```python
from build123d import *

# Parameters (mm, degrees)
BOSS_EXTRUDE1_DEPTH                    = 44
CBORE_FOR_M8_HEX_HEAD_BOLT1_AT_2_COUNT = 2
CBORE_FOR_M8_HEX_HEAD_BOLT1_AT_2_PITCH = 52
CBORE_FOR_M8_HEX_HEAD_BOLT1_AT_3_COUNT = 2
CBORE_FOR_M8_HEX_HEAD_BOLT1_AT_3_PITCH = 71.4177849
CBORE_FOR_M8_HEX_HEAD_BOLT1_AT_4_COUNT = 2
CBORE_FOR_M8_HEX_HEAD_BOLT1_AT_4_PITCH = 101
CBORE_FOR_M8_HEX_HEAD_BOLT1_AT_5_COUNT = 2
CBORE_FOR_M8_HEX_HEAD_BOLT1_AT_5_PITCH = 86.585218138
CBORE_FOR_M8_HEX_HEAD_BOLT1_AT_6_COUNT = 2
CBORE_FOR_M8_HEX_HEAD_BOLT1_AT_6_PITCH = 71.4177849
SKETCH9_W                              = 236.92276851
SKETCH9_H                              = 228.212372608
CUT_EXTRUDE1_DEPTH                     = 10
SKETCH8_R                              = 6
CUT_EXTRUDE2_DEPTH                     = 139.585713549


with BuildPart() as part:
    # Sketch1 → Boss-Extrude1 (new body)
    with BuildSketch(Plane(origin=(0, 0, 0), x_dir=(1, 0, 0), z_dir=(0, 1, 0))):
        with BuildLine():
            Line((77.338541491, -95), (-77.338541491, -95))
            ThreePointArc((-77.338541491, -95), (-86.620580695, -86.620580695), (-95, -77.338541491))
            Line((-95, -77.338541491), (-95, 77.338541491))
            ThreePointArc((-95, 77.338541491), (-86.620580695, 86.620580695), (-77.338541491, 95))
            Line((-77.338541491, 95), (77.338541491, 95))
            ThreePointArc((77.338541491, 95), (86.620580695, 86.620580695), (95, 77.338541491))
            Line((95, 77.338541491), (95, -77.338541491))
            ThreePointArc((95, -77.338541491), (86.620580695, -86.620580695), (77.338541491, -95))
        make_face()
    extrude(amount=BOSS_EXTRUDE1_DEPTH)

    # Sketch2 → Cut-Revolve3 (revolve, cut)
    with BuildSketch(Plane(origin=(0, 0, 0), x_dir=(0, 0, -1), z_dir=(1, 0, 0))):
        Polygon((90, 0), (90, 10), (60, 10), (60, 16.5), (41, 16.5), (41, 44), (0, 44), (0, 0), align=None)
    revolve(axis=Axis((0, 0, 0), (0, 1, 0)), mode=Mode.SUBTRACT)

    # Sketch3 → Cut-Revolve6 (revolve, cut)
    with BuildSketch(Plane(origin=(0, 0, 0), x_dir=(0, 0, -1), z_dir=(1, 0, 0))):
        Polygon((132.5, 25), (62.5, 25), (62.5, 35), (56.5, 41.8), (45, 41.8), (45, 44), (132.5, 44), align=None)
    revolve(axis=Axis((0, 0, 0), (0, 1, 0)), mode=Mode.SUBTRACT)

    # Sketch7 → CBORE for M8 Hex Head Bolt1 (revolve, cut)
    with BuildSketch(Plane(origin=(26, 16.5, -43.292609069), x_dir=(0, 0, -1), z_dir=(1, 0, 0))):
        Polygon((0, 0), (0, 27.5), (4.5, 27.5), (4.5, 13.025), (4.525, 13), (6.5, 13), (6.5, 0), align=None)
    cbore_for_m8_hex_head_bolt1 = revolve(axis=Axis((26, 10.15, -43.292609069), (0, 1, 0)), mode=Mode.SUBTRACT)

    # CBORE for M8 Hex Head Bolt1 at 2: CBORE for M8 Hex Head Bolt1 ×2
    with Locations(*[(-i * CBORE_FOR_M8_HEX_HEAD_BOLT1_AT_2_PITCH, 0, 0) for i in range(1, CBORE_FOR_M8_HEX_HEAD_BOLT1_AT_2_COUNT)]):
        add(cbore_for_m8_hex_head_bolt1, mode=Mode.SUBTRACT)

    # CBORE for M8 Hex Head Bolt1 at 3: CBORE for M8 Hex Head Bolt1 ×2
    with Locations(*[Vector(-0.9702430447284767, 0, 0.24213309182351622) * (i * CBORE_FOR_M8_HEX_HEAD_BOLT1_AT_3_PITCH) for i in range(1, CBORE_FOR_M8_HEX_HEAD_BOLT1_AT_3_COUNT)]):
        add(cbore_for_m8_hex_head_bolt1, mode=Mode.SUBTRACT)

    # CBORE for M8 Hex Head Bolt1 at 4: CBORE for M8 Hex Head Bolt1 ×2
    with Locations(*[Vector(-0.514851485148515, 0, 0.8572793875046621) * (i * CBORE_FOR_M8_HEX_HEAD_BOLT1_AT_4_PITCH) for i in range(1, CBORE_FOR_M8_HEX_HEAD_BOLT1_AT_4_COUNT)]):
        add(cbore_for_m8_hex_head_bolt1, mode=Mode.SUBTRACT)

    # CBORE for M8 Hex Head Bolt1 at 5: CBORE for M8 Hex Head Bolt1 ×2
    with Locations(*[(0, 0, i * CBORE_FOR_M8_HEX_HEAD_BOLT1_AT_5_PITCH) for i in range(1, CBORE_FOR_M8_HEX_HEAD_BOLT1_AT_5_COUNT)]):
        add(cbore_for_m8_hex_head_bolt1, mode=Mode.SUBTRACT)

    # CBORE for M8 Hex Head Bolt1 at 6: CBORE for M8 Hex Head Bolt1 ×2
    with Locations(*[Vector(0.24213309182351628, 0, 0.9702430447284767) * (i * CBORE_FOR_M8_HEX_HEAD_BOLT1_AT_6_PITCH) for i in range(1, CBORE_FOR_M8_HEX_HEAD_BOLT1_AT_6_COUNT)]):
        add(cbore_for_m8_hex_head_bolt1, mode=Mode.SUBTRACT)

    # Sketch9 → Cut-Extrude1 (cut)
    with BuildSketch(Plane.XZ.offset(-10)):
        Rectangle(SKETCH9_W, SKETCH9_H)
    extrude(amount=CUT_EXTRUDE1_DEPTH, mode=Mode.SUBTRACT)

    # Sketch8 → Cut-Extrude2 (cut, through all)
    with BuildSketch(Plane.XZ.offset(-10)):
        with Locations(Location((76.013978978, 76.013978978, 0), (0, 0, 270))):
            Circle(SKETCH8_R)
        with Locations(Location((81.915204429, 57.357643635, 0), (0, 0, 270))):
            Circle(SKETCH8_R)
        with Locations(Location((76.013978978, -76.013978978, 0), (0, 0, 270))):
            Circle(SKETCH8_R)
        with Locations(Location((57.357643635, -81.915204429, 0), (0, 0, 270))):
            Circle(SKETCH8_R)
        with Locations(Location((-76.013978978, -76.013978978, 0), (0, 0, 270))):
            Circle(SKETCH8_R)
        with Locations(Location((-81.915204429, -57.357643635, 0), (0, 0, 270))):
            Circle(SKETCH8_R)
        with Locations(Location((-76.013978978, 76.013978978, 0), (0, 0, 270))):
            Circle(SKETCH8_R)
        with Locations(Location((-57.357643635, 81.915204429, 0), (0, 0, 270))):
            Circle(SKETCH8_R)
    extrude(amount=-CUT_EXTRUDE2_DEPTH, mode=Mode.SUBTRACT)


solid = part.part
```
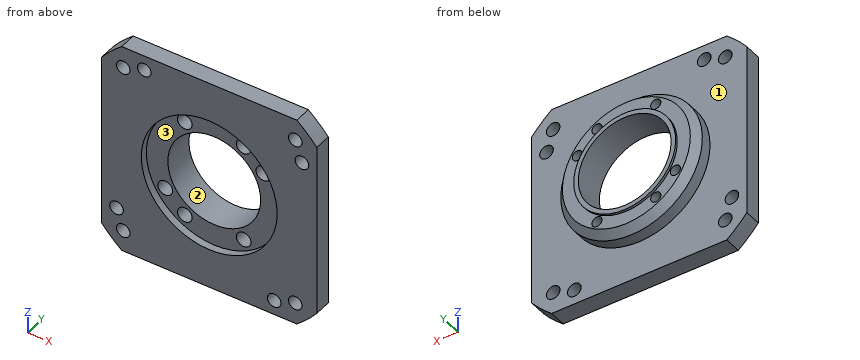
CAD build for the part. Positions are in the model's coordinates, mm. Face numbers are marked on the shaded views. Give positions to 0.01 mm unless a question says otherwise; leave off trailing zeros. Write each loop counter-clockwise with the first axis right and the second up, starting at its lowest first coordinate (ties: lowest second). Pieces come first, ordered by that corner, then holes. Notation, with made-up numbers: (48.5, 87.25) -> (62.5, 87.25) arc R19 cw to (62.5, 124.25) -> close; hole circle Ø7 at (28, 12). An arc over 180 degrees is marked (long way). Write each question's results on one line, items separated by ' | '.
1. Drop flat-ended pins along their axis: P1, Ø11.5, axis at x = -43.29, z = -26, coming from the -Y side; P2, Ø7, axis at x = 57.36, z = -81.92, coming from the -Y side; P3, Ø10.5, axis at x = -26, z = 40.5, coming from the -Y side; P4, Ø3, axis at y = 33, z = -55, coming from the +X side. Give the stop position or say it passes through.
Geometry check:
P1: y = 29.5 | P2: through | P3: y = 16.5 | P4: x = 32.31
2. Cut at C-C, the plane y = 32. Write the cut outline in (x, z), then the cut area to 3 significant figures.
Geometry check:
outline: circle Ø125 at (0, 0); hole circle Ø9 at (-43.29, -26); hole circle Ø82 at (0, 0); hole circle Ø9 at (-26, -43.29); hole circle Ø9 at (-26, 43.29); hole circle Ø9 at (26, -43.29); hole circle Ø9 at (26, 43.29); hole circle Ø9 at (43.29, 26) | area: 6,610 mm²
3. Cut at B-B, the plane z = 0. Write the cut outline in (x, y), then the cut area to 3 significant figures.
Geometry check:
outline: (-95, 10) -> (-60, 10) -> (-60, 16.5) -> (-41, 16.5) -> (-41, 44) -> (-45, 44) -> (-45, 41.8) -> (-56.5, 41.8) -> (-62.5, 35) -> (-62.5, 25) -> (-95, 25) -> close; (41, 16.5) -> (60, 16.5) -> (60, 10) -> (95, 10) -> (95, 25) -> (62.5, 25) -> (62.5, 35) -> (56.5, 41.8) -> (45, 41.8) -> (45, 44) -> (41, 44) -> close | area: 2,070 mm²
4. Wall check: probe 1 along X at (y, z) = (23, 57.5); probe 2 along X at (y, z) = (21.5, -27); probe 3 along X at (y, z) = (22, -28). Give the ranges that are in metal, low to high. Write a range as [from, to].
Geometry check:
probe 1: [-95, 75.92], [87.91, 95] | probe 2: [-95, -49.72], [-36.87, -30.85], [30.85, 95] | probe 3: [-95, -49.48], [-37.11, -29.95], [29.95, 95]
5. Cut at D-D, the plane z = 24.5. Give the number of separate pieces and of enclosed holes in the cut face, then the cut area to 3 significant figures.
Geometry check:
separate pieces: 3 | enclosed holes: 0 | area: 2,110 mm²
6. Two-plate mould, pull along Z, no slides. Class the marked faces 1, 2 and 3: pulls with the +Z half, pulls with the -Z half, needs draft (parallel to the pull), parting line crosses it, or undercut.
Geometry check:
face 1: needs draft | face 2: undercut | face 3: undercut
7. Cut at A-A, the plane x = 0. Write the cut outline in (y, z).
Geometry check:
outline: (10, -95) -> (25, -95) -> (25, -62.5) -> (35, -62.5) -> (41.8, -56.5) -> (41.8, -45) -> (44, -45) -> (44, -41) -> (16.5, -41) -> (16.5, -60) -> (10, -60) -> close; (10, 60) -> (16.5, 60) -> (16.5, 41) -> (44, 41) -> (44, 45) -> (41.8, 45) -> (41.8, 56.5) -> (35, 62.5) -> (25, 62.5) -> (25, 95) -> (10, 95) -> close
